The listing builds one solid part. Answer for the finished solid, in the listing's coordinates (mm). Round coordinates to 2 decimals unless told otherwise and drop trailing zeros. Write each loop counter-clockwise with the first axis right and the second up, starting at its lowest first coordinate (ties: lowest second). Pieces come first, ordered by that corner, then holes.
(1) A cutting plane is placed at A-A, the plane y = 89. Give the vertices of the cut face in (x, z), and give its area (3 significant figures).
(2) Each of these flat-tipped pins is pushed along its axis until it touches: pin 1 Ø1 at (x, y) = (1, 137) entering from +Z; pin 2 Ø1.2 at (x, y) = (0, 145.415) entering from -Z; pin 3 Ø1.6 at (y, z) = (147, 0) entering from +X. Where does it stop, or does it pass through?
(3) A cutting plane is placed at B-B, the plane z = 2.75. Give the vertices of the cut face in (x, y).
(4) Find the intervals of material crossed by probe 1 along Y at (x, z) = (0, 0.2); probe 2 along Y at (x, z) = (0.25, -0.5); probe 3 along Y at (x, z) = (-1.5, -1.25), in increasing order.
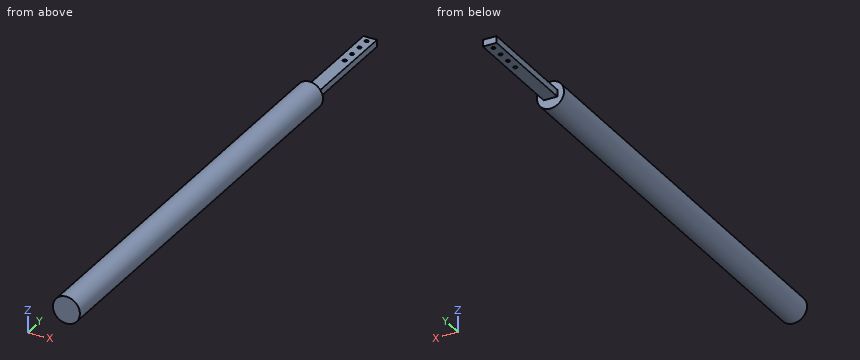
from build123d import *

# Parameters (mm, degrees)
SKETCH1_R           = 3.9624
BOSS_EXTRUDE1_DEPTH = 127
SKETCH4_W           = 4.000000128
SKETCH4_H           = 2
BOSS_EXTRUDE2_DEPTH = 31.75
SKETCH5_R           = 0.5334
CUT_EXTRUDE1_DEPTH  = 2


with BuildPart() as part:
    # Sketch1 → Boss-Extrude1 (new body)
    with BuildSketch(Plane(origin=(0, 0, 0), x_dir=(1, 0, 0), z_dir=(0, 1, 0))):
        with Locations(Location((0, 0, 0), (0, 0, 270))):
            Circle(SKETCH1_R)
    extrude(amount=BOSS_EXTRUDE1_DEPTH)

    # Sketch4 → Boss-Extrude2 (add)
    with BuildSketch(Plane(origin=(0, 127, 0), x_dir=(1, 0, 0), z_dir=(0, 1, 0))):
        with Locations((6.4e-08, 0)):
            Rectangle(SKETCH4_W, SKETCH4_H)
    extrude(amount=BOSS_EXTRUDE2_DEPTH)

    # Sketch5 → Cut-Extrude1 (cut)
    with BuildSketch(Plane(origin=(0, 0, -1), x_dir=(-1, 0, 0), z_dir=(0, 0, -1))):
        with Locations((0, 156.845)):
            Circle(SKETCH5_R)
        with Locations((0, 153.035)):
            Circle(SKETCH5_R)
        with Locations((0, 149.225)):
            Circle(SKETCH5_R)
        with Locations((0, 145.415)):
            Circle(SKETCH5_R)
    extrude(amount=-CUT_EXTRUDE1_DEPTH, mode=Mode.SUBTRACT)


solid = part.part
Solutions:
1. outline: circle Ø7.92 at (0, 0)
1. area: 49.3 mm2
2. pin 1: stops at z = 1
2. pin 2: stops at z = -1
2. pin 3: stops at x = 2
3. outline: (-2.85, 0) - (2.85, 0) - (2.85, 127) - (-2.85, 127) - close
4. probe 1: y = 0 to 144.88, 145.95 to 148.69, 149.76 to 152.5, 153.57 to 156.31, 157.38 to 158.75
4. probe 2: y = 0 to 144.94, 145.89 to 148.75, 149.7 to 152.56, 153.51 to 156.37, 157.32 to 158.75
4. probe 3: y = 0 to 127
